The listing builds one solid part. Answer for the finished solid, in the listing's coordinates (mm). Face numbers are marked on the shaded views. A direction names the side the tool comes from. Give positions to 0.01 mm unless a question says otherwise; leave off trailing zeros. Order: outer loops, then holes, each group sorted by start corner. A loop starts at its lowest first (then second) coordinate and runs counter-clockwise, first axis right, second up. Notation, with made-up numbers: (67, 77) - (107, 77) arc R20 ccw to (107, 104) - close; hole circle Ø7 at (52.25, 17). An arc over 180 degrees is marked (long way). Use a Markdown table: item, result. Add a question column.
1) Find section D-D, the plane x = -7. Determine the outline of the cut face in (y, z).
2) Flat-ended cylindrical pins translate along their axes: pin 1 (1.8 mm diameter, centred on x = 0, y = 0, fed in from +Z); pin 2 (1 mm diameter, centred on y = 17.5, z = 2, fed in from +X). Find the tip coordinate at first contact, or state that the pin passes through.
3) The mould has two halves that part along Y. Classify the marked faces 1, 2 and 3: released by +Y, released by -Y, zero draft, split by the parting line, or undercut.
4) Straight lines are drawn through the part: line 1 (Y direction, x = 0, z = 2.3); line 2 (Y direction, x = 13, z = 1.9); line 3 (X direction, y = 0, z = 1.25). For each, find the intervals that lie inside material, in ascending order.
5) Find section A-A, the plane x = 0. Determine the outline of the cut face in (y, z).
6) Find section B-B, the plane z = 1. Determine the outline of the cut face in (x, y), plus the area to 3 significant figures.
7) For the marked faces 4, 5, 6, 7 and 8, determine the directions among +Z, -Z, +X, -X, +Y, -Y from which every point of the face is accessible in a straight line to the end or side of a thin tool.
8) Find section C-C, the plane y = 0. Determine the outline of the cut face in (x, z), plus the area to 3 significant figures.
Autodesk Inventor part; units mm, degrees
ref_plane "YZ Plane" through (0, 0, 0) normal (1, 0, 0) x (0, 1, 0)
ref_plane "XZ Plane" through (0, 0, 0) normal (0, 1, 0) x (-1, 0, 0)
ref_plane "XY Plane" through (0, 0, 0) normal (0, 0, 1) x (1, 0, 0)
sketch "Sketch1" plane through (0, 0, 0) normal (0, 0, 1) x (1, 0, 0)
  circle A0 centre (0, 0) radius 10
  dimension "d0" = 20
extrude "Extrusion1" add sketch "Sketch1" along normal blind 3
sketch "Sketch2" plane through (0, 0, 3) normal (0, 0, 1) x (1, 0, 0)
  point P0 (0, 0)
  point P1 (0, 0)
hole "Hole1" at (0, 0, 3) direction (0, 0, -1) diameter 3 end through all
sketch "Sketch4" plane through (0, 0, 3) normal (0, 0, 1) x (1, 0, 0)
  circle A0 centre (0, 0) radius 10
  circle A1 centre (0, 20) radius 2.5
  circle A2 centre (0, 0) radius 1.5
  circle A3 centre (0, 0) radius 5
  line L0 (-4.9608, 0.625) -> (-2.4804, 20.3125)
  line L1 (2.4804, 20.3125) -> (4.9608, 0.625)
  dimension "d17" = 20
  dimension "d25" = 5
  dimension "d26" = 20
  dimension "d27" = 10
extrude "Extrusion2" add sketch "Sketch4" against normal up to surface (3 mm away) contours L1 A3 L0 A0 | A0 L0 A1 L1 | A1 picked at (-0.6594, 8.2675)
pattern_circular "Circular Pattern1" count 5 over 360 about axis through (0, 0, -10) along (0, 0, 1) of "Extrusion2"
properties part number "Selection_Gear 1" material "Nylon 6/6"
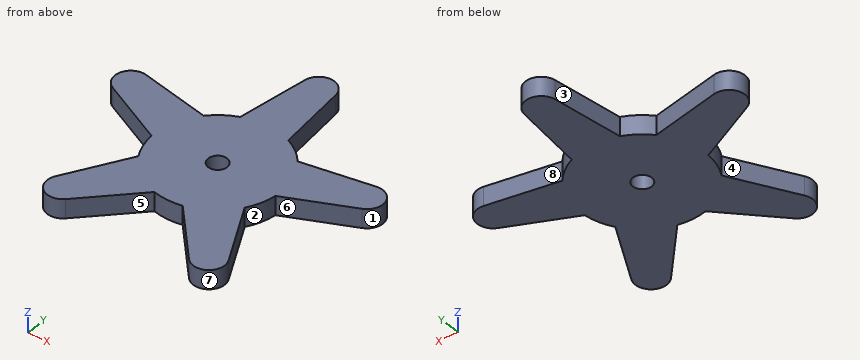
The answers:
| question | item | result |
|---|---|---|
| 1 | outline | (-14.77, 0) - (7.14, 0) - (7.14, 3) - (-14.77, 3) - close |
| 2 | pin 1 | through |
| 2 | pin 2 | x = 2.9 |
| 3 | face 1 | split by the parting line |
| 3 | face 2 | undercut |
| 3 | face 3 | released by +Y |
| 4 | line 1 | -10 to -1.5, 1.5 to 22.5 |
| 4 | line 2 | -18.35 to -13.26, 0.59 to 7.57 |
| 4 | line 3 | -11.75 to -1.5, 1.5 to 11.75 |
| 5 | outline | (-10, 0) - (-1.5, 0) - (-1.5, 3) - (-10, 3) - close; (1.5, 0) - (22.5, 0) - (22.5, 3) - (1.5, 3) - close |
| 6 | outline | (-20.08, 3.92) - (-9.96, -0.84) arc R10 ccw to (-8.56, -5.18) - (-13.95, -14.98) arc R2.5 ccw to (-9.93, -17.89) - (-2.28, -9.74) arc R10 ccw to (2.28, -9.74) - (9.93, -17.89) arc R2.5 ccw to (13.95, -14.98) - (8.56, -5.18) arc R10 ccw to (9.96, -0.84) - (20.08, 3.92) arc R2.5 ccw to (18.55, 8.64) - (7.57, 6.54) arc R10 ccw to (3.88, 9.22) - (2.48, 20.31) arc R2.5 ccw to (-2.48, 20.31) - (-3.88, 9.22) arc R10 ccw to (-7.57, 6.54) - (-18.55, 8.64) arc R2.5 ccw to start; hole circle Ø3 at (0, 0) |
| 6 | area | 681 mm2 |
| 7 | face 4 | +Z, -Z, -X |
| 7 | face 5 | +Z, -Z, -Y |
| 7 | face 6 | +Z, -Z, +X |
| 7 | face 7 | +Z, -Z |
| 7 | face 8 | +Z, -Z, +Y |
| 8 | outline | (-11.75, 0) - (-1.5, 0) - (-1.5, 3) - (-11.75, 3) - close; (1.5, 0) - (11.75, 0) - (11.75, 3) - (1.5, 3) - close |
| 8 | area | 61.5 mm2 |
